Read the model definition and answer for the solid it produces. Units are mm, in the model's axes. A direction names the side the tool comes from. Coordinates: 2 decimals unless noted, no trailing zeros. Loops run counter-clockwise (first coordinate to the right, second up) from the corner with the lowest first, then second, coordinate; pieces in that order, holes last. Notation, with made-up numbers: M -34.75,62.5 L 15.25,62.5 A17 cw 15.25,94.5 Z; hole C -15.5,-32.5 d5. An arc over 180 degrees is marked long. One line per item, written item: value. Start each with the question number.
```python
from build123d import *

# Parameters (mm, degrees)
EXTRUDE_1_DEPTH      = 15
EXTRUDE_2_DEPTH      = 15
EXTRUDE_3_DEPTH      = 13
EXTRUDE_4_DEPTH      = 10
CUT_EXTRUDE_2_DEPTH  = 43.818428432
CUT_EXTRUDE_3_DEPTH  = 10
EXTRUDE_5_DEPTH      = 13
EXTRUDE_5_DEPTH_BACK = 10
SKETCH_7_W           = 9.36410038
SKETCH_7_H           = 3.199645584
FILLET_1_R           = 1
SKETCH_8_R           = 2.377718278
CUT_EXTRUDE_4_DEPTH  = 1


with BuildPart() as part:
    # ｽｹｯﾁ1 → ﾎﾞｽ - 押し出し1 (new body)
    with BuildSketch(Plane.XY):
        with BuildLine():
            Line((5, 0), (15.5, 0))
            ThreePointArc((15.5, 0), (19.035533906, 1.464466094), (20.5, 5))
            Line((20.5, 5), (20.5, 11))
            ThreePointArc((20.5, 11), (19.035533906, 14.535533906), (15.5, 16))
            Line((15.5, 16), (5, 16))
            ThreePointArc((5, 16), (1.464466094, 14.535533906), (0, 11))
            Line((0, 11), (0, 5))
            ThreePointArc((0, 5), (1.464466094, 1.464466094), (5, 0))
        make_face()
    extrude(amount=EXTRUDE_1_DEPTH)

    # ｽｹｯﾁ2 → ﾎﾞｽ - 押し出し2 (add)
    with BuildSketch(Plane.XY.offset(15)):
        with BuildLine():
            ThreePointArc((10.25, 7.645751311), (3.25, 5), (10.25, 2.354248689))
            ThreePointArc((10.25, 2.354248689), (17.25, 5), (10.25, 7.645751311))
        make_face()
    extrude(amount=EXTRUDE_2_DEPTH)

    # ｽｹｯﾁ3 → ﾎﾞｽ - 押し出し3 (add)
    with BuildSketch(Plane.XY.offset(15)):
        Polygon((5, 8.307189139), (3.015149344, 10.292039795), (3.015149344, 15.589157643), (3.760031936, 15.843808337), (3.760031936, 10.292039795), (5.469966234, 8.582105497), align=None)
        Polygon((15.5, 8.307189139), (15.030033766, 8.582105497), (16.739968064, 10.292039795), (16.739968064, 15.843808337), (17.484850656, 15.589157643), (17.484850656, 10.292039795), align=None)
    extrude(amount=EXTRUDE_3_DEPTH)

    # ｽｹｯﾁ4 → ﾎﾞｽ - 押し出し4 (add)
    with BuildSketch(Plane(origin=(0, 0, 0), x_dir=(-1, 0, 0), z_dir=(0, 0, -1))):
        with BuildLine():
            Line((-19.035533906, 14.535533906), (-16.508167917, 20.778897002))
            ThreePointArc((-16.508167917, 20.778897002), (-15.404115105, 22.140884029), (-13.727372471, 22.653207574))
            Line((-13.727372471, 22.653207574), (-6.772627529, 22.653207574))
            ThreePointArc((-6.772627529, 22.653207574), (-5.095884895, 22.140884029), (-3.991832083, 20.778897002))
            Line((-3.991832083, 20.778897002), (-1.464466094, 14.535533906))
            Line((-1.464466094, 14.535533906), (-19.035533906, 14.535533906))
        make_face()
    extrude(amount=-EXTRUDE_4_DEPTH)

    # ｽｹｯﾁ5 → ｶｯﾄ - 押し出し2 (cut, through all)
    with BuildSketch(Plane(origin=(0, 0, 0), x_dir=(0, 0, -1), z_dir=(1, 0, 0))):
        Polygon((-10, 16), (-7.328208582, 22.653207574), (-10, 22.653207574), align=None)
    extrude(amount=CUT_EXTRUDE_2_DEPTH, mode=Mode.SUBTRACT)

    # ｽｹｯﾁ6 → ｶｯﾄ - 押し出し3 (cut)
    with BuildSketch(Plane(origin=(0, 0, 0), x_dir=(-1, 0, 0), z_dir=(0, 0, -1))):
        with BuildLine():
            Line((-14.93205019, 14.761085745), (-14.93205019, 20.248440553))
            ThreePointArc((-14.93205019, 20.248440553), (-14.639156971, 20.955547334), (-13.93205019, 21.248440553))
            Line((-13.93205019, 21.248440553), (-6.56794981, 21.248440553))
            ThreePointArc((-6.56794981, 21.248440553), (-5.860843029, 20.955547334), (-5.56794981, 20.248440553))
            Line((-5.56794981, 20.248440553), (-5.56794981, 14.761085745))
            add(Edge.make_bspline(
                [(-2.310743979, 13.961064345), (-3.233908529, 14.632656192), (-4.458845113, 14.799104366), (-5.56794981, 14.761085745)],
                knots=[0, 0, 0, 0, 1, 1, 1, 1], degree=3))
            ThreePointArc((-2.310743979, 13.961064345), (-1.342335165, 12.619100972), (-1, 11))
            Line((-1, 11), (-1, 5))
            ThreePointArc((-1, 5), (-2.171572875, 2.171572875), (-5, 1))
            Line((-5, 1), (-15.5, 1))
            ThreePointArc((-15.5, 1), (-18.328427125, 2.171572875), (-19.5, 5))
            Line((-19.5, 5), (-19.5, 11))
            ThreePointArc((-19.5, 11), (-19.157664835, 12.619100972), (-18.189256021, 13.961064345))
            add(Edge.make_bspline(
                [(-18.189256021, 13.961064345), (-17.266091471, 14.632656192), (-16.041154887, 14.799104366), (-14.93205019, 14.761085745)],
                knots=[0, 0, 0, 0, 1, 1, 1, 1], degree=3))
        make_face()
    extrude(amount=-CUT_EXTRUDE_3_DEPTH, mode=Mode.SUBTRACT)

    # ｽｹｯﾁ7 → ﾎﾞｽ - 押し出し5 (add, two sides: drawn at the far end of the back side and taken through both)
    with BuildSketch(Plane.XY.offset(15).offset(-EXTRUDE_5_DEPTH_BACK)):
        with Locations((10.25, 15.098663031)):
            Rectangle(SKETCH_7_W, SKETCH_7_H)
    extrude(amount=EXTRUDE_5_DEPTH + EXTRUDE_5_DEPTH_BACK)

    # ﾌｨﾚｯﾄ1
    # the kernel refuses this fillet: 1 mm, written as the material it takes off along each edge
    with BuildSketch(Plane(origin=(14.93205019, 16.698485823, 5), x_dir=(0, 0, 1), z_dir=(-1, 0, 0))) as fillet_1_piece_1:
        with BuildLine():
            CenterArc((FILLET_1_R, -FILLET_1_R), FILLET_1_R, 90, 90)
            Line((0, -FILLET_1_R), (0, 0))
            Line((0, 0), (FILLET_1_R, 0))
        make_face()
    extrude(amount=9.36410038, mode=Mode.SUBTRACT)
    with BuildSketch(Plane(origin=(14.93205019, 13.498840239, 2.5), x_dir=(0, 1, 0), z_dir=(0, 0, 1))) as fillet_1_piece_2:
        with BuildLine():
            CenterArc((FILLET_1_R, FILLET_1_R), FILLET_1_R, 180, 90)
            Line((0, FILLET_1_R), (0, 0))
            Line((0, 0), (FILLET_1_R, 0))
        make_face()
    extrude(amount=7.5, mode=Mode.SUBTRACT)
    with BuildSketch(Plane(origin=(5.56794981, 13.498840239, 2.5), x_dir=(0, 1, 0), z_dir=(0, 0, 1))) as fillet_1_piece_3:
        with BuildLine():
            CenterArc((FILLET_1_R, -FILLET_1_R), FILLET_1_R, 90, 90)
            Line((0, -FILLET_1_R), (0, 0))
            Line((0, 0), (FILLET_1_R, 0))
        make_face()
    extrude(amount=7.5, mode=Mode.SUBTRACT)
    with BuildSketch(Plane(origin=(5.56794981, 13.498840239, 15), x_dir=(0, 1, 0), z_dir=(0, 0, 1)), Plane(origin=(14.93205019, 13.498840239, 15), x_dir=(-1, 0, 0), z_dir=(0, 0, 1))) as fillet_1_piece_4:
        with BuildLine():
            CenterArc((FILLET_1_R, -FILLET_1_R), FILLET_1_R, 90, 90)
            Line((0, -FILLET_1_R), (0, 0))
            Line((0, 0), (FILLET_1_R, 0))
        make_face()
    extrude(amount=15.5, mode=Mode.SUBTRACT)
    with BuildSketch(Plane(origin=(14.93205019, 16.698485823, 30.5), x_dir=(0, -1, 0), z_dir=(0, 0, -1))) as fillet_1_piece_5_section:
        with BuildLine():
            CenterArc((FILLET_1_R, FILLET_1_R), FILLET_1_R, 180, 90)
            Line((0, FILLET_1_R), (0, 0))
            Line((0, 0), (FILLET_1_R, 0))
        make_face()
    fillet_1_piece_5 = extrude(amount=23.280497551, mode=Mode.PRIVATE)
    fillet_1_piece_5 = split(fillet_1_piece_5, bisect_by=Plane(origin=(14.918146213, 15.92497671, 15), z_dir=(0, 0, 1)), keep=Keep.TOP, mode=Mode.PRIVATE)
    add(fillet_1_piece_5, mode=Mode.SUBTRACT)
    with BuildSketch(Plane(origin=(14.93205019, 16.698485823, 30.5), x_dir=(0, -1, 0), z_dir=(0, 0, -1))) as fillet_1_piece_6_section:
        with BuildLine():
            CenterArc((FILLET_1_R, FILLET_1_R), FILLET_1_R, 180, 90)
            Line((0, FILLET_1_R), (0, 0))
            Line((0, 0), (FILLET_1_R, 0))
        make_face()
    fillet_1_piece_6 = extrude(amount=23.280497551, mode=Mode.PRIVATE)
    fillet_1_piece_6 = split(fillet_1_piece_6, bisect_by=Plane(origin=(14.70262804, 15.590982586, 10.164252987), z_dir=(0, 0.3726538497201509, 0.927970424253247)), keep=Keep.TOP, mode=Mode.PRIVATE)
    fillet_1_piece_6 = split(fillet_1_piece_6, bisect_by=Plane(origin=(14.70262804, 16, 12.401713298), z_dir=(0, 1, 0)), keep=Keep.TOP, mode=Mode.PRIVATE)
    add(fillet_1_piece_6, mode=Mode.SUBTRACT)
    with BuildSketch(Plane(origin=(5.56794981, 16.698485823, 30.5), x_dir=(0, -1, 0), z_dir=(0, 0, -1))) as fillet_1_piece_7_section:
        with BuildLine():
            CenterArc((FILLET_1_R, -FILLET_1_R), FILLET_1_R, 90, 90)
            Line((0, -FILLET_1_R), (0, 0))
            Line((0, 0), (FILLET_1_R, 0))
        make_face()
    fillet_1_piece_7 = extrude(amount=23.280497551, mode=Mode.PRIVATE)
    fillet_1_piece_7 = split(fillet_1_piece_7, bisect_by=Plane(origin=(5.581853787, 15.92497671, 15), z_dir=(0, 0, 1)), keep=Keep.TOP, mode=Mode.PRIVATE)
    add(fillet_1_piece_7, mode=Mode.SUBTRACT)
    with BuildSketch(Plane(origin=(5.56794981, 16.698485823, 30.5), x_dir=(0, -1, 0), z_dir=(0, 0, -1))) as fillet_1_piece_8_section:
        with BuildLine():
            CenterArc((FILLET_1_R, -FILLET_1_R), FILLET_1_R, 90, 90)
            Line((0, -FILLET_1_R), (0, 0))
            Line((0, 0), (FILLET_1_R, 0))
        make_face()
    fillet_1_piece_8 = extrude(amount=23.280497551, mode=Mode.PRIVATE)
    fillet_1_piece_8 = split(fillet_1_piece_8, bisect_by=Plane(origin=(5.79737196, 16, 12.401713298), z_dir=(0, 1, 0)), keep=Keep.TOP, mode=Mode.PRIVATE)
    fillet_1_piece_8 = split(fillet_1_piece_8, bisect_by=Plane(origin=(5.79737196, 15.590982586, 10.164252987), z_dir=(0, 0.3726538497201509, 0.927970424253247)), keep=Keep.TOP, mode=Mode.PRIVATE)
    add(fillet_1_piece_8, mode=Mode.SUBTRACT)

    # ｽｹｯﾁ8 → ｶｯﾄ - 押し出し4 (cut)
    with BuildSketch(Plane.XY.offset(30)):
        with Locations((10.235322727, 5.074085352)):
            Circle(SKETCH_8_R)
    extrude(amount=-CUT_EXTRUDE_4_DEPTH, mode=Mode.SUBTRACT)


solid = part.part
```
1) Section D-D (z = 26) is taken. Determine the outline of the cut face in (x, y), then the cut area to 3 significant figures.
2) Consider line 1 along X through (y, z) = (15.5, 26); line 2 along X through (y, z) = (12, 27); line 3 along X through (y, z) = (6.75, 4.5). Determine where each line is inside the solid, lowest interval first.
3) Section C-C (z = 11) is taken. Determine the outline of the cut face in (x, y).
4) A tool of negligible diameter and unlimited length cuts with its end or side. For faces 1 (the face through (14.932, 15, 21)), 2 (the face through (10, 15, 28)), 3 (the face through (10, 13.499, 21)), 4 (the face through (5.568, 18, 4)), 5 (the face through (17.485, 13, 21)), from which of +Z, -Z, +X, -X, +Y, -Y can it reach the whole face along a straight path? Write none if from no direction.
5) For a pull along Y with two mould halves and no side action, classify faces 6 (the face through (19.63, 13.82, 9.06)), 7 (the face through (14.647, 20.948, 4.089)), 8 (the face through (10, 8, 10)), 9 (the face through (5.568, 15, 21)) as released by +Y, released by -Y, zero draft, split by the parting line, or undercut.
6) Section B-B (y = 18.5) is taken. Determine the outline of the cut face in (x, z), then the cut area to 3 significant figures.
7) Section A-A (x = 13.25) is taken. Determine the outline of the cut face in (y, z).
8) Flat-ended cylindrical pins translate along their axes: pin 1 (6 mm diameter, centred on x = 9.5, z = 24.5, fed in from +Y); pin 2 (1.2 mm diameter, centred on x = 17, y = 15.5, fed in from +Z); pin 3 (6 mm diameter, centred on y = 16, z = 4, fed in from +X). Find the tip coordinate at first contact, or state that the pin passes through.
Results found:
1. outline: M 3.02,10.29 L 5,8.31 A4 ccw long 10.25,2.35 A4 ccw long 15.5,8.31 L 17.48,10.29 L 17.48,15.59 L 16.74,15.84 L 16.74,10.29 L 15.03,8.58 A4 ccw 10.25,7.65 A4 ccw 5.47,8.58 L 3.76,10.29 L 3.76,15.84 L 3.02,15.59 Z; M 5.57,14.5 A1 ccw 6.57,13.5 L 13.93,13.5 A1 ccw 14.93,14.5 L 14.93,15.7 A1 ccw 13.93,16.7 L 6.57,16.7 A1 ccw 5.57,15.7 Z
1. area: 133 mm²
2. line 1: x = 3.02 to 3.76, 5.57 to 14.93, 16.74 to 17.48
2. line 2: x = 3.02 to 3.76, 16.74 to 17.48
2. line 3: x = 0 to 1, 19.5 to 20.5
3. outline: M 0,5 A5 ccw 5,0 L 15.5,0 A5 ccw 20.5,5 L 20.5,11 A5 ccw 15.5,16 L 14.89,16 A1 ccw 13.93,16.7 L 6.57,16.7 A1 ccw 5.61,16 L 5,16 A5 ccw 0,11 Z
4. face 1: +Z, +Y
4. face 2: +Z, +X, -X, +Y
4. face 3: +Z
4. face 4: -Z
4. face 5: +Z, +X, +Y, -Y
5. face 6: released by +Y
5. face 7: undercut
5. face 8: undercut
5. face 9: zero draft
6. outline: M 3.07,0 L 5.57,0 L 5.57,9 L 3.07,9 Z; M 14.93,0 L 17.43,0 L 17.43,9 L 14.93,9 Z
6. area: 45.0 mm²
7. outline: M 0,0 L 1,0 L 1,10 L 13.5,10 L 13.5,5 L 15.7,5 A1 ccw 16.7,6 L 16.7,28 L 13.5,28 L 13.5,15 L 9,15 L 9,30 L 1,30 L 1,15 L 0,15 Z; M 21.25,0 L 22.65,0 L 22.65,7.33 L 21.25,7.89 Z
8. pin 1: stops at y = 16.7
8. pin 2: stops at z = 28
8. pin 3: stops at x = 20.08
